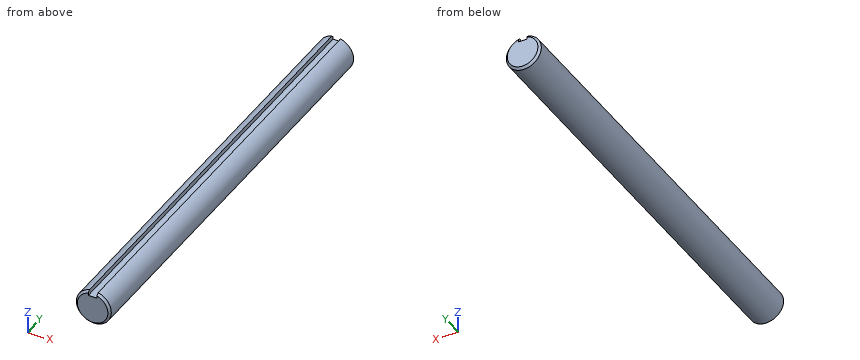
```python
from build123d import *

# Parameters (mm, degrees)
SKETCH1_R           = 4
BOSS_EXTRUDE1_DEPTH = 100
SKETCH2_W           = 2
SKETCH2_H           = 2
CUT_EXTRUDE1_DEPTH  = 101.159872204
CHAMFER1_SIZE       = 0.5


with BuildPart() as part:
    # Sketch1 → Boss-Extrude1 (new body)
    with BuildSketch(Plane(origin=(0, 0, 0), x_dir=(1, 0, 0), z_dir=(0, 1, 0))):
        with Locations(Location((0, 0, 0), (0, 0, 270))):
            Circle(SKETCH1_R)
    extrude(amount=BOSS_EXTRUDE1_DEPTH)

    # Sketch2 → Cut-Extrude1 (cut, through all)
    with BuildSketch(Plane.XZ):
        with Locations((0, 3.8)):
            Rectangle(SKETCH2_W, SKETCH2_H)
    extrude(amount=-CUT_EXTRUDE1_DEPTH, mode=Mode.SUBTRACT)

    # Chamfer1
    chamfer1_edges = [part.edges().sort_by_distance(p)[0] for p in [
        (0, 0, -4),
        (0, 100, -4),
    ]]
    chamfer(chamfer1_edges, length=CHAMFER1_SIZE)


solid = part.part
```
Check sheet for the modelled part. Datum: model origin and axes. Units: mm. Give positions to 0.01 mm unless a question says otherwise; leave off trailing zeros. Order: outer loops, then holes, each group sorted by start corner. A loop starts at its lowest first (then second) coordinate and runs counter-clockwise, first axis right, second up. Notation, with made-up numbers: M 59.25,89 L 85.25,89 A12 cw 85.25,96 Z; hole C -1.75,73.25 d1. An arc over 180 degrees is marked long. Answer in a Markdown table with one row per item. Add a question column.
Q1. Thickness scan on L1, parallel to X at y = 24, z = 3; L2, parallel to X at y = 7, z = 3.5; L3, parallel to Z at x = -0.25, y = 93.5. Record the ranges inside material, lowest first.
Q2. Sectioned sample at B-B, the plane y = 65.5. Record the boundary of the cut face in (x, z).
Q3. Gauge pin test, flat ends, axial feed: pin 1 Ø0.9 at (y, z) = (26, 3.5) entering from +X; pin 2 Ø1 at (x, y) = (0, 62) entering from +Z; pin 3 Ø2 at (y, z) = (48.5, -3) entering from +X. Record the tip position at first contact, or that the pin passes through.
Q4. Sectioned sample at A-A, the plane x = 0. Record the boundary of the cut face in (y, z), and give its area (3 significant figures).
Verdict:
| question | item | result |
|---|---|---|
| 1 | L1 | -2.65 to -1, 1 to 2.65 |
| 1 | L2 | -1.94 to -1, 1 to 1.94 |
| 1 | L3 | -3.99 to 2.8 |
| 2 | outline | M -1,2.8 L -1,3.87 A4 ccw long 1,3.87 L 1,2.8 Z |
| 3 | pin 1 | x = 2.59 |
| 3 | pin 2 | z = 2.8 |
| 3 | pin 3 | x = 3.46 |
| 4 | outline | M 0,-3.5 L 0.5,-4 L 99.5,-4 L 100,-3.5 L 100,2.8 L 0,2.8 Z |
| 4 | area | 680 mm² |
